from build123d import *

# Parameters (mm, degrees)
CYLINDER054_R          = 2.5
CYLINDER054_DEPTH      = 30
CYLINDER053_R          = 4
CYLINDER053_DEPTH      = 30
CUT056_PLACEMENT_ANGLE = 25


with BuildPart() as cylinder054:
    # Cylinder054 → Cylinder054 (new body)
    with BuildSketch(Plane.XY):
        Circle(CYLINDER054_R)
    extrude(amount=CYLINDER054_DEPTH)


with BuildPart() as obj1:
    # Cylinder053 → Cylinder053 (new body)
    with BuildSketch(Plane.XY):
        Circle(CYLINDER053_R)
    extrude(amount=CYLINDER053_DEPTH)

    # Cut056: cut Cylinder054
    add(cylinder054.part, mode=Mode.SUBTRACT)


with BuildPart() as obj1_1:
    # Cut056 placement: moved
    add(obj1.part.moved(Location((-1.218022, 50.6, -43.017699))).rotate(Axis((-1.218022, 50.6, -43.017699), (0, 1, 0)), CUT056_PLACEMENT_ANGLE))


solid = obj1_1.part
Can you work these out from the model? Positions are in its coordinate system, mm. Give positions to 0.01 mm unless a question says otherwise; leave off trailing zeros. Order: outer loops, then holes, each group sorted by start corner. A loop starts at its lowest first (then second) coordinate and runs counter-clockwise, first axis right, second up. Notation, with made-up numbers: M 63,-36 L 93,-36 A28 ccw 93,-8 Z; hole C 50,-32.5 d5. An arc over 180 degrees is marked long. Use a Markdown table: item, result. Add a question column.
Item 1: Will these pins go through, and if not, where does the flat tip stop? pin 1 (1.5 mm diameter, centred on y = 53, z = -36.5, fed in from +X); pin 2 (2 mm diameter, centred on y = 53, z = -40.5, fed in from +X); pin 3 (1.5 mm diameter, centred on y = 51.5, z = -28, fed in from +X).
Item 2: Suppose I cut it at C-C (y = 47.75). List the corners of the cut face in (x, z) for me.
Item 3: Suppose I cut it at D-D (y = 53.5). List the corners of the cut face in (x, z) for me.
Item 4: Suppose I cut it at B-B (y = 51.75). List the corners of the cut face in (x, z) for me, then the cut area to 3 significant figures.
Item 5: If I drill on L1, parallel to X at y = 51, z = -17; L2, parallel to Y at x = 3.5, z = -37; L3, parallel to Z at x = 7.5, y = 50.75, over which ranges is the centre line in solid material (lowest first)? Write a range as [from, to].
Item 6: Suppose I cut it at A-A (y = 49.5). List the corners of the cut face in (x, z) for me, then the cut area to 3 significant figures.
Item 7: We'd pull the mould along X, two halves only. Please class faces 1 (the flat face through (1.1, 49.8, -44.1)), 2 (the flat face through (13.827, 49.767, -16.932)), 3 (the cylindrical face through (4.54, 48.16, -29.38)): +X half, -X half, draft (parallel to the pull), parting line (faces both ways), or undercut.
Answer sheet:
| question | item | result |
|---|---|---|
| 1 | pin 1 | stops at x = 5.97 |
| 1 | pin 2 | stops at x = 4.29 |
| 1 | pin 3 | stops at x = 10.47 |
| 2 | outline | M -3.76,-41.83 L 1.33,-44.2 L 14,-17.01 L 8.92,-14.64 Z |
| 3 | outline | M -3.71,-41.85 L 1.28,-44.18 L 13.96,-16.99 L 8.96,-14.66 Z |
| 4 | outline | M -4.69,-41.4 L -3.23,-42.08 L 9.45,-14.89 L 7.99,-14.21 Z; M 0.79,-43.96 L 2.25,-44.64 L 14.93,-17.45 L 13.47,-16.77 Z |
| 4 | area | 96.7 mm² |
| 5 | L1 | x = [6.52, 8.19], [13.64, 13.97] |
| 5 | L2 | y = [46.99, 48.8], [52.4, 54.21] |
| 5 | L3 | z = [-33.78, -30.23], [-18.42, -14.86] |
| 6 | outline | M -4.7,-41.39 L -3.25,-42.07 L 9.43,-14.88 L 7.98,-14.2 Z; M 0.82,-43.97 L 2.27,-44.64 L 14.95,-17.45 L 13.5,-16.78 Z |
| 6 | area | 96.0 mm² |
| 7 | face 1 | -X half |
| 7 | face 2 | +X half |
| 7 | face 3 | undercut |
